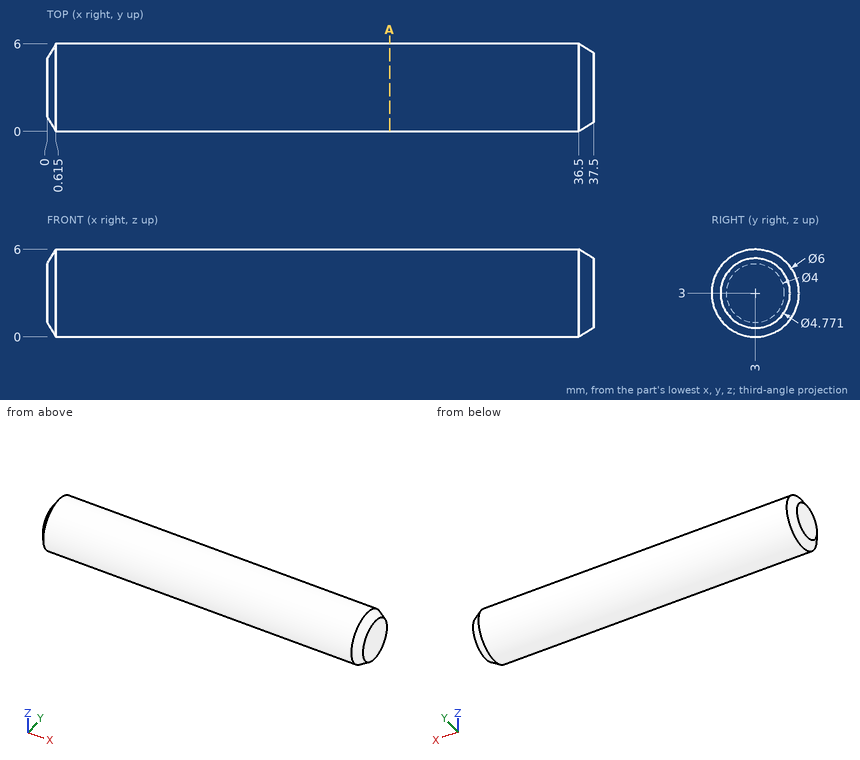
For this review, use the dimensioned drawing (mm, ordinates from the lowest corner) and the shaded views. Coordinates: 2 decimals unless noted, no trailing zeros. Order: outer loops, then holes, each group sorted by start corner. A loop starts at its lowest first (then second) coordinate and runs counter-clockwise, first axis right, second up. Notation, with made-up numbers: (28.5, 30) - (40.5, 30) arc R18 ccw to (40.5, 51) - close; hole circle Ø7 at (5, 73.5). An arc over 180 degrees is marked (long way). Answer as a JSON object with one key per item and string values. Group by question number.
1. For probe 1 along Z at (x, y) = (10, 3.2); probe 2 along Z at (x, y) = (14, 0.55) (1 decimal); probe 3 along Y at (x, z) = (23.5, 3.3) (1 decimal), list the stretches that pass through material, from the lowest coordinate up.
2. Clearance check with a flat-ended pin moving along its axis: P1, Ø1.5, axis at x = 18.5, z = 5.5, coming from the -Y side. State where the tip first meets the part, or that it passes through.
3. We need section A-A on x = 23.5. State the section outline as (y, z) points.
Final values:
{
 "1": {"probe 1": "0.01 to 5.99", "probe 2": "1.3 to 4.7", "probe 3": "0 to 6"},
 "2": {"P1": "y = 0.56"},
 "3": {"outline": "circle Ø6 at (3, 3)"}
}
